```python
from build123d import *

# Parameters (mm, degrees)
SKETCH1_R           = 3.3655
BOSS_EXTRUDE1_DEPTH = 86.91372
FILLET1_R           = 3.3655


with BuildPart() as part:
    # Sketch1 → Boss-Extrude1 (new body)
    with BuildSketch(Plane(origin=(0, 0, 0), x_dir=(1, 0, 0), z_dir=(0, 1, 0))):
        with Locations(Location((0, 0, 0), (0, 0, 270))):
            Circle(SKETCH1_R)
    extrude(amount=BOSS_EXTRUDE1_DEPTH)

    # Sketch2 → Cut-Revolve2 (revolve, cut)
    with BuildSketch(Plane(origin=(48.790895882, 11.267332823, -12.664317923), x_dir=(0.9679254058512238, 0, -0.2512377533487826), z_dir=(0.2512377533487826, 0, 0.9679254058512238)), mode=Mode.PRIVATE) as cut_revolve2_sk:
        with BuildLine():
            Line((-53.773202481, 66.327127177), (-53.376327481, 66.327127177))
            ThreePointArc((-53.376327481, 66.327127177), (-52.815061473, 66.094643184), (-52.582577481, 65.533377177))
            Line((-52.582577481, 65.533377177), (-52.582577481, 64.671534192))
            ThreePointArc((-52.582577481, 64.671534192), (-52.642998102, 64.367779217), (-52.815061473, 64.110268184))
            Line((-52.815061473, 64.110268184), (-53.773202481, 63.152127177))
            Line((-53.773202481, 63.152127177), (-53.773202481, 66.327127177))
        make_face()
    revolve(cut_revolve2_sk.sketch.rotate(Axis((0, 86.91372, 0), (0, -1, 0)), 14.550768137), axis=Axis((0, 86.91372, 0), (0, -1, 0)), mode=Mode.SUBTRACT)

    # Fillet1
    fillet1_edges = [part.edges().sort_by_distance(p)[0] for p in [
        (0, 86.91372, -3.3655),
    ]]
    fillet(fillet1_edges, radius=FILLET1_R)


solid = part.part
```
Here's how the part is built. I have some questions about the finished solid (model axes, mm). A direction names the side the tool comes from. Give positions to 0.01 mm unless a question says otherwise; leave off trailing zeros. Order: outer loops, then holes, each group sorted by start corner. A loop starts at its lowest first (then second) coordinate and runs counter-clockwise, first axis right, second up. Notation, with made-up numbers: (-30, 55.5) - (2, 55.5) arc R17 cw to (2, 75.5) - close; hole circle Ø8 at (-6, 53.25). An arc over 180 degrees is marked (long way). Answer as a JSON object with one key per item and string values. Group by question number.
Item 1: If we section it at C-C on y = 27: Please give me the cut outline in (x, z).
Item 2: If we section it at A-A on z = 0: Please give me the cut outline in (x, y), and give its area (3 significant figures).
Item 3: If we section it at B-B on x = 0: Please give me the cut outline in (y, z).
Item 4: For P1, Ø2, axis at y = 17.5, z = 2, coming from the +X side; P2, Ø2, axis at y = 37, z = -1.5, coming from the +X side, each with a flat end and sliding along its axis, tell me the tip position at first contact or that it passes through.
Item 5: Please list where these lines run through material, in increasing order: probe 1 along X at (y, z) = (36, -0.25); probe 2 along Y at (x, z) = (1, -2.25).
Item 6: Which directions (+Z, -Z, +X, -X, +Y, -Y) give clear straight access to the entire face, cutting with the end or side of a thin tool? Please do faces 1 (the flat face through (-1, 77.594, 3)), 2 (the cylindrical face through (-1.29, 80.53, 3.11)).
Item 7: If we mould it in two halves opening along Y, with no side actions, what happens to faces 3 (the cylindrical face through (1.603, 76.364, -1.47)), 4 (the flat face through (0, 0, 0)), 5 (the cylindrical face through (-1.29, 36.69, 3.11))? For each: pulls with the +Y half, pulls with the -Y half, needs draft (parallel to the pull), parting line crosses it, or undercut.
Result set:
{
 "1": {"outline": "circle Ø6.73 at (0, 0)"},
 "2": {"outline": "(-3.37, 0) - (3.37, 0) - (3.37, 74.42) - (2.41, 75.38) arc R0.79 cw to (2.17, 75.94) - (2.17, 76.8) arc R0.79 cw to (2.97, 77.59) - (3.37, 77.59) - (3.37, 83.55) arc R3.37 ccw to (-3.37, 83.55) - (-3.37, 77.59) - (-2.97, 77.59) arc R0.79 cw to (-2.17, 76.8) - (-2.17, 75.94) arc R0.79 cw to (-2.41, 75.38) - (-3.37, 74.42) - close", "area": "574 mm²"},
 "3": {"outline": "(0, -3.37) - (74.42, -3.37) - (75.38, -2.41) arc R0.79 cw to (75.94, -2.17) - (76.8, -2.17) arc R0.79 cw to (77.59, -2.97) - (77.59, -3.37) - (83.55, -3.37) arc R3.37 ccw to (83.55, 3.37) - (77.59, 3.37) - (77.59, 2.97) arc R0.79 cw to (76.8, 2.17) - (75.94, 2.17) arc R0.79 cw to (75.38, 2.41) - (74.42, 3.37) - (0, 3.37) - close"},
 "4": {"P1": "x = 3.21", "P2": "x = 3.33"},
 "5": {"probe 1": "-3.36 to 3.36", "probe 2": "0 to 75.32, 77.41 to 85.84"},
 "6": {"face 1": "none", "face 2": "+Y, -Y"},
 "7": {"face 3": "undercut", "face 4": "pulls with the -Y half", "face 5": "needs draft"}
}
